```python
from build123d import *

# Parameters (mm, degrees)
SKETCH1_R               = 11
BOSS_EXTRUDE1_DEPTH     = 3.5
CUT_EXTRUDE3_REACH      = 46.858
CUT_EXTRUDE3_END_RADIUS = 13
SKETCH2_W               = 8
SKETCH2_H               = 3
CIRPATTERN1_COUNT       = 8


with BuildPart() as part:
    # Sketch1 → Boss-Extrude1 (new, symmetric)
    with BuildSketch(Plane.XY):
        Polygon((8.284271247, 20), (-8.284271247, 20), (-20, 8.284271247), (-20, -8.284271247), (-8.284271247, -20), (8.284271247, -20), (20, -8.284271247), (20, 8.284271247), align=None)
        Circle(SKETCH1_R, mode=Mode.SUBTRACT)
    extrude(amount=BOSS_EXTRUDE1_DEPTH, both=True)

    # Cut-Extrude3: up to this cylinder (the profile starts outside it)
    cut_extrude3_end = Plane(origin=(0, 0, 0), z_dir=(0, 0, -1)) * Cylinder(CUT_EXTRUDE3_END_RADIUS, 120.716, mode=Mode.PRIVATE)
    # Sketch2 → Cut-Extrude3 (cut, up to the surface)
    with BuildSketch(Plane(origin=(0, -20, 0), x_dir=(-1, 0, 0), z_dir=(0, -1, 0)), mode=Mode.PRIVATE) as cut_extrude3_sk1:
        Rectangle(SKETCH2_W, SKETCH2_H)
    cut_extrude3_tool1 = extrude(cut_extrude3_sk1.sketch, amount=-CUT_EXTRUDE3_REACH, mode=Mode.PRIVATE) - cut_extrude3_end
    cut_extrude3 = cut_extrude3_tool1.solids().sort_by_distance((0, -20, 0))[0]
    add(cut_extrude3, mode=Mode.SUBTRACT)

    # CirPattern1: Cut-Extrude3 ×8 about axis
    cirpattern1_axis = Axis((0, 0, 0), (0, 0, 1))
    for i in range(1, CIRPATTERN1_COUNT):
        add(cut_extrude3.rotate(cirpattern1_axis, i * 360 / CIRPATTERN1_COUNT), mode=Mode.SUBTRACT)


solid = part.part
```
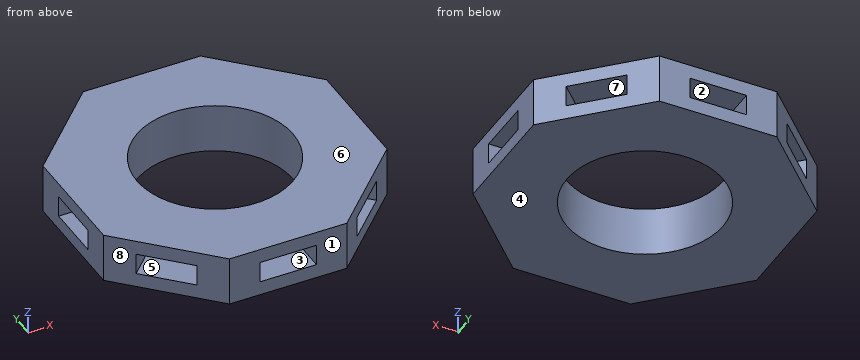
Build history of the part. All positions in model axes, mm. Face numbers are marked on the shaded views. A direction names the side the tool comes from. Round coordinates to 2 decimals unless told otherwise and drop trailing zeros. Order: outer loops, then holes, each group sorted by start corner. A loop starts at its lowest first (then second) coordinate and runs counter-clockwise, first axis right, second up. Notation, with made-up numbers: (74.5, -11) -> (92.5, -11) arc R38 cw to (92.5, 28) -> close; hole circle Ø4 at (-12.75, 82.5). An arc over 180 degrees is marked (long way). Answer in a Markdown table with one row per item.
1) Pin check, flat tips, straight feed: P1, Ø6, axis at x = 9, y = 0.5, coming from the -Z side; P2, Ø0.9, axis at y = 17, z = -0.5, coming from the -X side; P3, Ø1.5, axis at y = -13, z = -2, coming from the -X side; P4, Ø2.5, axis at y = -17, z = -0.5, coming from the -X side. Stop position of each tip, or through.
Values:
| item | result |
|---|---|
| P1 | z = -3.5 |
| P2 | x = -11.31 |
| P3 | x = -16.03 |
| P4 | x = -12.03 |
2) Mould opens along Z. For the marked faces 6, 7 and 8 say: released by +Z, released by -Z, zero draft, split by the parting line, or undercut.
Values:
| item | result |
|---|---|
| face 6 | released by +Z |
| face 7 | undercut |
| face 8 | zero draft |
3) Band-saw the part on C-C on z = -2.5. Give the cut face in (x, y).
Values:
| item | result |
|---|---|
| outline | (-20, -8.28) -> (-8.28, -20) -> (8.28, -20) -> (20, -8.28) -> (20, 8.28) -> (8.28, 20) -> (-8.28, 20) -> (-20, 8.28) -> close; hole circle Ø22 at (0, 0) |
4) Which spindle directions (+Z, -Z, +X, -X, +Y, -Y) get a long thin tool onto all of the face, cutting with end or side? Do the marked faces 1, 2, 3, 4 and 5. Say none if no direction does.
Values:
| item | result |
|---|---|
| face 1 | +Z, -Z, +X, -X, -Y |
| face 2 | +Y |
| face 3 | -Y |
| face 4 | -Z, +X, -X, +Y, -Y |
| face 5 | none |
5) Wall check: L1, parallel to Z at x = -12.5, y = 11.5; L2, parallel to Y at x = 0, z = -0.5; L3, parallel to Y at x = 8, z = 2. Give the ranges that are in metal, low to high.
Values:
| item | result |
|---|---|
| L1 | -3.5 to -1.5, 1.5 to 3.5 |
| L2 | -13 to -11, 11 to 13 |
| L3 | -20 to -7.55, 7.55 to 20 |
6) Band-saw the part on A-A on y = 0. Give the cut face in (x, z), and give its area (3 significant figures).
Values:
| item | result |
|---|---|
| outline | (-20, -3.5) -> (-11, -3.5) -> (-11, 3.5) -> (-20, 3.5) -> (-20, 1.5) -> (-13, 1.5) -> (-13, -1.5) -> (-20, -1.5) -> close; (11, -3.5) -> (20, -3.5) -> (20, -1.5) -> (13, -1.5) -> (13, 1.5) -> (20, 1.5) -> (20, 3.5) -> (11, 3.5) -> close |
| area | 84.0 mm2 |
7) Band-saw the part on D-D on y = 17.5. Give the cut face in (x, z), and give its area (3 significant figures).
Values:
| item | result |
|---|---|
| outline | (-10.78, -3.5) -> (10.78, -3.5) -> (10.78, 3.5) -> (-10.78, 3.5) -> close; hole (-4, -1.5) -> (4, -1.5) -> (4, 1.5) -> (-4, 1.5) -> close |
| area | 127 mm2 |
